Geometry: final body of the model. Coordinates: model frame, mm. A direction names the side the tool comes from. Coordinates: 2 decimals unless noted, no trailing zeros. Write each loop counter-clockwise with the first axis right and the second up, starting at its lowest first coordinate (ties: lowest second). Pieces come first, ordered by that corner, then holes. Notation, with made-up numbers: M 38,57 L 67,57 A17 ccw 67,88 Z; hole C 60,57.25 d5. An arc over 180 degrees is marked long. Write item = value, one per line. Start each with the question number.
Item 1: First-contact query: pin 1 Ø1.5 at (y, z) = (4.5, 17) entering from -X; pin 2 Ø6 at (x, y) = (9, 8) entering from +Z; pin 3 Ø2 at (x, z) = (-27.5, 22) entering from +Y. Flat tips, straight axial feed; report the tip coordinate or a pass-through.
Item 2: Pull-direction query (X, two-part tool) for faces 1 (the flat face through (1, 17.5, 2)), 2 (the cylindrical face through (48.5, -16.07, 1.97)), 3 (the cylindrical face through (-48.57, -16, 1.97)), 4 (the cylindrical face through (-14.96, -3.8, 15.83)); classes: +X half, -X half, draft (parallel to the pull), parting line (faces both ways), or undercut.
Item 3: Ray query, L1, parallel to Z at x = 10.5, y = 7; L2, parallel to X at y = 3, z = 23.75; L3, parallel to Y at x = 12.5, z = 23.25. Return the intervals inside material, ascending. Write a range as [from, to].
Item 4: Section B-B on y = 0. Output: boundary loops of the cut face in (x, z).
Item 5: Section A-A on x = -10. Output: boundary loops of the cut face in (y, z), plus the area to 3 significant figures.
Item 6: Reachability of faces 5 (the flat face through (50, 0, 2)), 6 (the cylindrical face through (15.96, 1.88, 15.83)) from +Z, -Z, +X, -X, +Y, -Y: full face, straight path, thin tool, end or side. Return the list, or none.
Item 7: Section C-C on z = 24.5. Output: boundary loops of the cut face in (x, y).
Item 8: Section D-D on x = 0.5. Output: boundary loops of the cut face in (y, z), plus the area to 3 significant figures.
from build123d import *

# Parameters (mm, degrees)
F0_R     = 6.25
F1_DEPTH = 30
F2_DEPTH = 4
F3_SIZE  = 2


with BuildPart() as f1:
    # F0 (on Top) → F1 (new body)
    with BuildSketch(Plane.XY):
        with Locations((-30, 0)):
            Circle(F0_R)
        with Locations((-10, 0)):
            Circle(F0_R)
        with Locations((10, 0)):
            Circle(F0_R)
        with Locations((30, 0)):
            Circle(F0_R)
    extrude(amount=F1_DEPTH)

    # F0 (on Top) → F2 (join)
    with BuildSketch(Plane.XY):
        with BuildLine():
            ThreePointArc((50, 12.5), (48.535534, 16.035534), (45, 17.5))
            Line((45, 17.5), (-45, 17.5))
            ThreePointArc((-45, 17.5), (-48.535534, 16.035534), (-50, 12.5))
            Line((-50, 12.5), (-50, -12.5))
            ThreePointArc((-50, -12.5), (-48.535534, -16.035534), (-45, -17.5))
            Line((-45, -17.5), (45, -17.5))
            ThreePointArc((45, -17.5), (48.535534, -16.035534), (50, -12.5))
            Line((50, -12.5), (50, 12.5))
        make_face()
        with Locations((-30, 0)):
            Circle(F0_R, mode=Mode.SUBTRACT)
        with Locations((-10, 0)):
            Circle(F0_R, mode=Mode.SUBTRACT)
        with Locations((10, 0)):
            Circle(F0_R, mode=Mode.SUBTRACT)
        with Locations((30, 0)):
            Circle(F0_R, mode=Mode.SUBTRACT)
    extrude(amount=F2_DEPTH)

    # F3
    f3_edges = [f1.edges().sort_by_distance(p)[0] for p in [
        (-36.25, 0, 30),
        (-16.25, 0, 30),
        (3.75, 0, 30),
        (23.75, 0, 30),
    ]]
    chamfer(f3_edges, length=F3_SIZE)


solid = f1.part
Responses:
q1.pin_1 = -35
q1.pin_2 = 29.19
q1.pin_3 = 6.07
q2.face_1 = draft
q2.face_2 = +X half
q2.face_3 = -X half
q2.face_4 = undercut
q3.L1 = [0, 4]
q3.L2 = [-35.48, -24.52], [-15.48, -4.52], [4.52, 15.48], [24.52, 35.48]
q3.L3 = [-5.73, 5.73]
q4.outline = M -50,0 L 50,0 L 50,4 L 36.25,4 L 36.25,28 L 34.25,30 L 25.75,30 L 23.75,28 L 23.75,4 L 16.25,4 L 16.25,28 L 14.25,30 L 5.75,30 L 3.75,28 L 3.75,4 L -3.75,4 L -3.75,28 L -5.75,30 L -14.25,30 L -16.25,28 L -16.25,4 L -23.75,4 L -23.75,28 L -25.75,30 L -34.25,30 L -36.25,28 L -36.25,4 L -50,4 Z
q5.outline = M -17.5,0 L 17.5,0 L 17.5,4 L 6.25,4 L 6.25,28 L 4.25,30 L -4.25,30 L -6.25,28 L -6.25,4 L -17.5,4 Z
q5.area = 461 mm²
q6.face_5 = +Z, -Z, +X, +Y, -Y
q6.face_6 = +Z
q7.outline = C -30,0 d12.5; C -10,0 d12.5; C 10,0 d12.5; C 30,0 d12.5
q8.outline = M -17.5,0 L 17.5,0 L 17.5,4 L -17.5,4 Z
q8.area = 140 mm²
